Could you check a few things on this model? Use its own coordinates, in mm. A direction names the side the tool comes from. Give positions to 0.01 mm unless a question says otherwise; leave off trailing zeros. Loops run counter-clockwise (first coordinate to the right, second up) from the corner with the lowest first, then second, coordinate; pieces in that order, holes last. Notation, with made-up numbers: (73.5, -16) -> (127.5, -16) arc R11 ccw to (127.5, -5) -> close; hole circle Ø9 at (57, 75.25). An arc over 180 degrees is marked (long way). Put each result on its own line as item: value.
```python
from build123d import *

# Parameters (mm, degrees)
BOSS_EXTRUDE1_DEPTH = 600
BOSS_EXTRUDE2_DEPTH = 63
BOSS_EXTRUDE4_DEPTH = 7
SKETCH10_R          = 6
CUT_EXTRUDE3_DEPTH  = 7
FILLET5_R           = 5


with BuildPart() as part:
    # Sketch1 → Boss-Extrude1 (new body)
    with BuildSketch(Plane.XY):
        Polygon((0, 0), (0, 70), (70, 70), (70, 63), (7, 63), (7, 0), align=None)
    extrude(amount=BOSS_EXTRUDE1_DEPTH)

    # Sketch2 → Boss-Extrude2 (add)
    with BuildSketch(Plane(origin=(0, 0, 0), x_dir=(1, 0, 0), z_dir=(0, 1, 0))):
        Polygon((0, -600), (25, -643.301270189), (31.062177826, -639.801270189), (7, -600), align=None)
    extrude(amount=BOSS_EXTRUDE2_DEPTH)

    # Sketch9 → Boss-Extrude4 (add)
    with BuildSketch(Plane(origin=(0, 63, 0), x_dir=(1, 0, 0), z_dir=(0, 1, 0))):
        with BuildLine():
            Line((0, -600), (25, -643.301270189))
            ThreePointArc((25, -643.301270189), (29.250444511, -646.562750973), (34.562177826, -645.863448016))
            Line((34.562177826, -645.863448016), (70, -625.403411844))
            Line((70, -625.403411844), (70, -600))
            Line((70, -600), (0, -600))
        make_face()
    extrude(amount=BOSS_EXTRUDE4_DEPTH)

    # Sketch10 → Cut-Extrude3 (cut)
    with BuildSketch(Plane(origin=(-260.517992164, 0, 157.498246278), x_dir=(-0.5173609804017633, 0, -0.8557672674026079), z_dir=(0.8557672674026079, 0, -0.5173609804017633))):
        with Locations((-538.591343444, 35)):
            Circle(SKETCH10_R)
    extrude(amount=-CUT_EXTRUDE3_DEPTH, mode=Mode.SUBTRACT)

    # Fillet5
    fillet5_edges = [part.edges().sort_by_distance(p)[0] for p in [
        (7, 63, 300),
        (19.031088913, 63, 619.900635095),
    ]]
    fillet(fillet5_edges, radius=FILLET5_R)

    # Mirror6: part across plane


with BuildPart() as part_1:
    add(part.part)
    add(part.part.mirror(Plane.XY))


solid = part_1.part
```
1. I'm going to push flat-ended pins straight in: pin 1 (1 mm diameter, centred on x = 35, z = -235, fed in from -Y); pin 2 (8 mm diameter, centred on y = 53, z = -172, fed in from -X); pin 3 (3 mm diameter, centred on y = 51, z = 85, fed in from +X). Where does each tip first touch, or does it pass through?
Recorded:
pin 1: stops at y = 63
pin 2: stops at x = 0
pin 3: stops at x = 7
2. If we section it at B-B (z = -523): List the corners of the cut face in (x, y) for me.
Recorded:
outline: (0, 0) -> (7, 0) -> (7, 58) arc R5 cw to (12, 63) -> (70, 63) -> (70, 70) -> (0, 70) -> close
3. If we section it at A-A (y = 11): List the corners of the cut face in (x, z) for me, then the cut area to 3 significant figures.
Recorded:
outline: (0, -600) -> (25, -643.3) -> (31.06, -639.8) -> (7, -600) -> (7, 600) -> (31.06, 639.8) -> (25, 643.3) -> (0, 600) -> close
area: 9,030 mm^2
4. For faces 1 (the face through (52.03, 66.45, 635.78)), 2 (the face through (19.2, 28.59, 620.18)), which set-ups out of +Z, -Z, +X, -X, +Y, -Y let a thin tool reach every point of the face, with its end or its side?
Recorded:
face 1: +Z, +X, +Y, -Y
face 2: +X, -Y
5. I need wall thicknesses on line 1 (Y direction, x = 59, z = -349.5); line 2 (X direction, y = 29, z = -96.5); line 3 (Z direction, x = 20, y = 5.5). Which ranges of each line are inside material? Lowest first, please.
Recorded:
line 1: y = 63 to 70
line 2: x = 0 to 7
line 3: z = -634.64 to -621.5, 621.5 to 634.64
